```python
from build123d import *

# Parameters (mm, degrees)
F0_R     = 30
F0_R_2   = 27.5
F1_DEPTH = 31
F0_R_3   = 25
F2_DEPTH = 1
F3_DEPTH = 30


with BuildPart() as f1:
    # F0 (on Front) → F1 (new body)
    with BuildSketch(Plane.XZ):
        Circle(F0_R)
        Circle(F0_R_2, mode=Mode.SUBTRACT)
    extrude(amount=F1_DEPTH)

    # F0 (on Front) → F2 (join)
    with BuildSketch(Plane.XZ):
        Circle(F0_R_2)
        Circle(F0_R_3, mode=Mode.SUBTRACT)
    extrude(amount=F2_DEPTH)

    # F0 (on Front) → F3 (join)
    with BuildSketch(Plane.XZ):
        Circle(F0_R)
        Circle(F0_R_2, mode=Mode.SUBTRACT)
    extrude(amount=-F3_DEPTH)


solid = f1.part
```
Input: part model. Units: mm. Frame: model coordinates. A direction names the side the tool comes from. Coordinates: 2 decimals unless noted, no trailing zeros. Write each loop counter-clockwise with the first axis right and the second up, starting at its lowest first coordinate (ties: lowest second). Pieces come first, ordered by that corner, then holes. Notation, with made-up numbers: (9, -37.5) -> (19, -37.5) arc R15 ccw to (19, -10.5) -> close; hole circle Ø6 at (8.5, 53.25). An arc over 180 degrees is marked (long way). Write each question's results on one line, items separated by ' | '.
Item 1: Set-up query: faces 1 (the cylindrical face through (-5.961, -15.79, -26.846)), 2 (the cylindrical face through (-5.961, 14.79, -26.846)), 3 (the cylindrical face through (23.846, -0.493, 7.509)). Return all of +Z, -Z, +X, -X, +Y, -Y with unobstructed straight access to the full face (end or side cutting, diameter ignored); none if empty.
Conclusion:
face 1: -Y | face 2: +Y | face 3: +Y, -Y
Item 2: Section query B-B on z = 0. Return loops of the section in (x, y), plus the area to 3 significant figures.
Conclusion:
outline: (-30, -31) -> (-27.5, -31) -> (-27.5, -1) -> (-25, -1) -> (-25, 0) -> (-27.5, 0) -> (-27.5, 30) -> (-30, 30) -> close; (25, -1) -> (27.5, -1) -> (27.5, -31) -> (30, -31) -> (30, 30) -> (27.5, 30) -> (27.5, 0) -> (25, 0) -> close | area: 310 mm^2
Item 3: Mould query, pull axis X, two halves, no side actions, for faces 4 (the cylindrical face through (-29.97, -0.93, 1.32)), 5 (the flat face through (12.1, 0, -22.3)), 6 (the flat face through (13.2, -31, -24.3)). Classes: +X half, -X half, draft (parallel to the pull), parting line (faces both ways), or undercut.
Conclusion:
face 4: parting line | face 5: undercut | face 6: draft
Item 4: Material intervals for probe 1 along Z at (x, y) = (0, -0.3); probe 2 along Z at (x, y) = (0, -13), sorted ascending.
Conclusion:
probe 1: z = -30 to -25, 25 to 30 | probe 2: z = -30 to -27.5, 27.5 to 30
Item 5: Section query C-C on y = 6.5. Return loops of the section in (x, z).
Conclusion:
outline: circle Ø60 at (0, 0); hole circle Ø55 at (0, 0)
Item 6: Pin query (flat end, axial travel): pin 1 Ø5 at (x, y) = (-23, -24.5) entering from -Z; pin 2 Ø8 at (x, y) = (-0.5, -9.5) entering from -Z; pin 3 Ø5 at (x, y) = (5.5, -24) entering from +Z. Return the tip coordinate at first contact, or that it passes through.
Conclusion:
pin 1: stops at z = -21.9 | pin 2: stops at z = -30 | pin 3: stops at z = 29.85
Item 7: Section query A-A on x = 0. Return loops of the section in (y, z), plus the area to 3 significant figures.
Conclusion:
outline: (-31, -30) -> (30, -30) -> (30, -27.5) -> (0, -27.5) -> (0, -25) -> (-1, -25) -> (-1, -27.5) -> (-31, -27.5) -> close; (-31, 27.5) -> (-1, 27.5) -> (-1, 25) -> (0, 25) -> (0, 27.5) -> (30, 27.5) -> (30, 30) -> (-31, 30) -> close | area: 310 mm^2
